Autodesk Inventor part; units mm, degrees
ref_plane "YZ Plane" through (0, 0, 0) normal (1, 0, 0) x (0, 1, 0)
ref_plane "XZ Plane" through (0, 0, 0) normal (0, 1, 0) x (-1, 0, 0)
ref_plane "XY Plane" through (0, 0, 0) normal (0, 0, 1) x (1, 0, 0)
sketch "Esboço1" plane through (0, 0, 0) normal (0, 1, 0) x (-1, 0, 0)
  circle A0 centre (0, 0) radius 40
  line L0 (-40, 0) -> (-40, -25.4828)
  line L1 (-40, -25.4828) -> (0.3313, -44.2896)
  line L2 (0.3313, -44.2896) -> (19.9786, -44.2896)
  line L3 (20.6627, -44.4102) -> (33.3415, -49.0249)
  line L4 (32.6574, -52.9043) -> (-40, -52.9043)
  arc A1 (32.6574, -52.9043) -> (33.3415, -49.0249) centre (32.6574, -50.9043) ccw
  arc A2 (20.6627, -44.4102) -> (19.9786, -44.2896) centre (19.9786, -46.2896) ccw
  line L5 (-40, -52) -> (32.6574, -52)
  arc A3 (32.6574, -52) -> (33.0322, -49.8747) centre (32.6574, -50.9043) ccw
  line L6 (33.0322, -49.8747) -> (20.3534, -45.26)
  arc A4 (20.3534, -45.26) -> (19.9786, -45.1939) centre (19.9786, -46.2896) ccw
  line L7 (19.9786, -45.1939) -> (0.1308, -45.1939)
  line L8 (0.1308, -45.1939) -> (-40.9043, -26.0589)
  line L9 (-40.9043, -26.0589) -> (-40.9043, 0)
  line L10 (-40, -52) -> (-40, -52.9043)
  line L11 (40, 0) -> (-40, 0)
  line L12 (-40, 0) -> (-40, 25.4828)
  line L13 (-40, 25.4828) -> (0.3313, 44.2896)
  line L14 (0.3313, 44.2896) -> (19.9786, 44.2896)
  line L15 (20.6627, 44.4102) -> (33.3415, 49.0249)
  line L16 (32.6574, 52.9043) -> (-40, 52.9043)
  arc A5 (33.3415, 49.0249) -> (32.6574, 52.9043) centre (32.6574, 50.9043) ccw
  arc A6 (19.9786, 44.2896) -> (20.6627, 44.4102) centre (19.9786, 46.2896) ccw
  line L17 (-40, 52) -> (32.6574, 52)
  arc A7 (33.0322, 49.8747) -> (32.6574, 52) centre (32.6574, 50.9043) ccw
  line L18 (33.0322, 49.8747) -> (20.3534, 45.26)
  arc A8 (19.9786, 45.1939) -> (20.3534, 45.26) centre (19.9786, 46.2896) ccw
  line L19 (19.9786, 45.1939) -> (0.1308, 45.1939)
  line L20 (0.1308, 45.1939) -> (-40.9043, 26.0589)
  line L21 (-40.9043, 26.0589) -> (-40.9043, 0)
  line L22 (-40, 52) -> (-40, 52.9043)
  point P0 (20.3313, -44.2896)
  dimension "d0" = 80
  dimension "d1" = 115
  dimension "d4" = 20
  dimension "d5" = 160
  dimension "d6" = 2
  dimension "d7" = 0.9043
  dimension "d8" = 7.7104
  dimension "d9" = 34.6649
  dimension "d10" = 20.6748
extrude "Extrusão1" add sketch "Esboço1" along normal blind 40 contours L13 L12 L0 L1 L2 A2 L3 A1 L4 L10 L5 A3 L6 A4 L7 L8 L9 L21 L20 L19 A8 L18 A7 L17 L22 L16 A5 L15 A6 L14
equation "\"Raio_dobra\" = Espessura"
equation "\"Largura_alívio_de_dobra\" = Espessura"
equation "\"Profundidade_alívio_de_dobra\" = 0.5 * Espessura"
equation "\"Tamanho_alívio_de_dobra\" = 4 * Espessura"
equation "\"Remanescente_mínimo\" = 2 * Espessura"
equation "\"Raiodetransição\" = Raio_dobra"
equation "\"Tamanho_de_raio_de_Jacobi\" = Raio_dobra"
equation "\"TamanhoFolga\" = Espessura"
properties part number "Garra"
Geometry check sheet. Reference: the model listing, model coordinates, mm. A direction names the side the tool comes from. Coordinates: 2 decimals unless noted, no trailing zeros. Order: outer loops, then holes, each group sorted by start corner. A loop starts at its lowest first (then second) coordinate and runs counter-clockwise, first axis right, second up. Notation, with made-up numbers: (65, 31.25) - (113, 31.25) arc R19 ccw to (113, 64.25) - close; hole circle Ø5 at (86, 79.5). An arc over 180 degrees is marked (long way). One line per item, written item: value.
(1) Release check for a two-part mould opening along Z. For faces 4 (the face through (-26.78, 19.72, 47.6)), 5 (the face through (28.5, 40, 31.6)), 6 (the face through (-33.74, 19.72, -51.07)), 7 (the face through (3, 20, 52.904)) record: +Z half, -Z half, draft (parallel to the pull), parting line (faces both ways), or undercut.
Data:
face 4: undercut
face 5: draft
face 6: undercut
face 7: +Z half
(2) Sectioned sample at A-A (x = -11). Enter the section's corners in (y, z), and give its area (3 significant figures).
Data:
outline: (0, -52.9) - (40, -52.9) - (40, -52) - (0, -52) - close; (0, -45.19) - (40, -45.19) - (40, -44.29) - (0, -44.29) - close; (0, 44.29) - (40, 44.29) - (40, 45.19) - (0, 45.19) - close; (0, 52) - (40, 52) - (40, 52.9) - (0, 52.9) - close
area: 145 mm^2
(3) Access from +Z, -Z, +X, -X, +Y, -Y to the whole of each face (thin tool, end or side, straight path). Record for faces 1 (the face through (4, 20, -52)), 2 (the face through (-26.913, 19.72, -46.685)), 3 (the face through (28.5, 0, 31.6)).
Data:
face 1: +X, +Y, -Y
face 2: -X, +Y, -Y
face 3: +Z, -Z, +X, -X, -Y
(4) Sectioned sample at C-C (z = 6). Enter the section's corners in (x, y), and give its area (3 significant figures).
Data:
outline: (40, 0) - (40.9, 0) - (40.9, 40) - (40, 40) - close
area: 36.2 mm^2
(5) Depth check by flat-ended pin: pin 1 Ø4 at (y, z) = (30, -21) entering from -X; pin 2 Ø6 at (x, z) = (17.5, 41.5) entering from -Y; pin 3 Ø0.5 at (y, z) = (19, 52.5) entering from +X. Enter the tip coordinate at first touch or a pass-through.
Data:
pin 1: stops at x = 40
pin 2: passes through
pin 3: stops at x = 40
(6) Sectioned sample at B-B (y = 15.5). Enter the section's corners in (x, z), and give its area (3 significant figures).
Data:
outline: (-33.34, -49.02) arc R2 ccw to (-32.66, -52.9) - (40, -52.9) - (40, -52) - (-32.66, -52) arc R1.1 cw to (-33.03, -49.87) - (-20.35, -45.26) arc R1.1 cw to (-19.98, -45.19) - (-0.13, -45.19) - (40.9, -26.06) - (40.9, 26.06) - (-0.13, 45.19) - (-19.98, 45.19) arc R1.1 cw to (-20.35, 45.26) - (-33.03, 49.87) arc R1.1 cw to (-32.66, 52) - (40, 52) - (40, 52.9) - (-32.66, 52.9) arc R2 ccw to (-33.34, 49.02) - (-20.66, 44.41) arc R2 ccw to (-19.98, 44.29) - (-0.33, 44.29) - (40, 25.48) - (40, -25.48) - (-0.33, -44.29) - (-19.98, -44.29) arc R2 ccw to (-20.66, -44.41) - close
area: 328 mm^2
(7) Sectioned sample at D-D (x = -23). Enter the section's corners in (y, z), and give its area (3 significant figures).
Data:
outline: (0, -52.9) - (40, -52.9) - (40, -52) - (0, -52) - close; (0, -46.22) - (40, -46.22) - (40, -45.26) - (0, -45.26) - close; (0, 45.26) - (40, 45.26) - (40, 46.22) - (0, 46.22) - close; (0, 52) - (40, 52) - (40, 52.9) - (0, 52.9) - close
area: 149 mm^2
(8) Thickness scan on probe 1 along Z at (x, y) = (-14, 6); probe 2 along Z at (x, y) = (-25, 30); probe 3 along X at (y, z) = (27.5, -2). Record the ranges inside material, lowest first. Write a range as from..to.
Data:
probe 1: z = -52.9..-52, -45.19..-44.29, 44.29..45.19, 52..52.9
probe 2: z = -52.9..-52, -46.95..-45.99, 45.99..46.95, 52..52.9
probe 3: x = 40..40.9
